from build123d import *

# Parameters (mm, degrees)
SKETCH_1_R          = 17
EXTRUDE_1_DEPTH     = 4
CUT_EXTRUDE_1_DEPTH = 2
CUT_EXTRUDE_2_REACH = 26.372
SKETCH_3_R          = 2
SKETCH_3_R_2        = 1
FILLET_1_R          = 1


with BuildPart() as part:
    # 草图1 → 凸台-拉伸1 (new body)
    with BuildSketch(Plane(origin=(0, 0, 0), x_dir=(1, 0, 0), z_dir=(0, 1, 0))):
        with Locations(Location((0, 0, 0), (0, 0, 270))):
            Circle(SKETCH_1_R)
    extrude(amount=EXTRUDE_1_DEPTH)

    # 草图2 → 切除-拉伸1 (cut)
    with BuildSketch(Plane(origin=(0, 0, 0), x_dir=(1, 0, 0), z_dir=(0, 1, 0))):
        with BuildLine():
            Line((2.5, 4.5), (2.5, -4.5))
            ThreePointArc((2.5, -4.5), (0, -7), (-2.5, -4.5))
            Line((-2.5, -4.5), (-2.5, 4.5))
            ThreePointArc((-2.5, 4.5), (0, 7), (2.5, 4.5))
        make_face()
    extrude(amount=CUT_EXTRUDE_1_DEPTH, mode=Mode.SUBTRACT)

    # 草图3 → 切除-拉伸2 (cut, up to next)
    with BuildSketch(Plane(origin=(0, 4, 0), x_dir=(1, 0, 0), z_dir=(0, 1, 0)), mode=Mode.PRIVATE) as cut_extrude_2_sk1:
        with Locations(Location((0, 11, 0), (0, 0, 270))):
            Circle(SKETCH_3_R)
    cut_extrude_2_tool1 = extrude(cut_extrude_2_sk1.sketch, amount=-CUT_EXTRUDE_2_REACH, mode=Mode.PRIVATE) & part.part
    # 草图3 → 切除-拉伸2 (cut, up to next)
    with BuildSketch(Plane(origin=(0, 4, 0), x_dir=(1, 0, 0), z_dir=(0, 1, 0)), mode=Mode.PRIVATE) as cut_extrude_2_sk2:
        with Locations(Location((-7.778174593, 7.778174593, 0), (0, 0, 270))):
            Circle(SKETCH_3_R_2)
    cut_extrude_2_tool2 = extrude(cut_extrude_2_sk2.sketch, amount=-CUT_EXTRUDE_2_REACH, mode=Mode.PRIVATE) & part.part
    # 草图3 → 切除-拉伸2 (cut, up to next)
    with BuildSketch(Plane(origin=(0, 4, 0), x_dir=(1, 0, 0), z_dir=(0, 1, 0)), mode=Mode.PRIVATE) as cut_extrude_2_sk3:
        with Locations(Location((11, 0, 0), (0, 0, 270))):
            Circle(SKETCH_3_R)
    cut_extrude_2_tool3 = extrude(cut_extrude_2_sk3.sketch, amount=-CUT_EXTRUDE_2_REACH, mode=Mode.PRIVATE) & part.part
    # 草图3 → 切除-拉伸2 (cut, up to next)
    with BuildSketch(Plane(origin=(0, 4, 0), x_dir=(1, 0, 0), z_dir=(0, 1, 0)), mode=Mode.PRIVATE) as cut_extrude_2_sk4:
        with Locations(Location((7.778174593, -7.778174593, 0), (0, 0, 270))):
            Circle(SKETCH_3_R_2)
    cut_extrude_2_tool4 = extrude(cut_extrude_2_sk4.sketch, amount=-CUT_EXTRUDE_2_REACH, mode=Mode.PRIVATE) & part.part
    add(cut_extrude_2_tool1.solids().sort_by_distance((0, 4, -11))[0], mode=Mode.SUBTRACT)
    add(cut_extrude_2_tool2.solids().sort_by_distance((-7.778175, 4, -7.778175))[0], mode=Mode.SUBTRACT)
    add(cut_extrude_2_tool3.solids().sort_by_distance((11, 4, 0))[0], mode=Mode.SUBTRACT)
    add(cut_extrude_2_tool4.solids().sort_by_distance((7.778175, 4, 7.778175))[0], mode=Mode.SUBTRACT)

    # 圆角1
    fillet_1_edges = [part.edges().sort_by_distance(p)[0] for p in [
        (0, 0, -17),
    ]]
    fillet(fillet_1_edges, radius=FILLET_1_R)


solid = part.part
Geometry check sheet. Reference: the model listing, model coordinates, mm. A direction names the side the tool comes from. Round coordinates to 2 decimals unless told otherwise and drop trailing zeros. Write each loop counter-clockwise with the first axis right and the second up, starting at its lowest first coordinate (ties: lowest second). Pieces come first, ordered by that corner, then holes. Notation, with made-up numbers: (-38, 86.25) -> (-8, 86.25) arc R20 ccw to (-8, 124.25) -> close; hole circle Ø8 at (66.25, -21). An arc over 180 degrees is marked (long way). One line per item, written item: value. Start each with the question number.
(1) Draft check along Z on faces 1 (the flat face through (0, 4, 0)), 2 (the cylindrical face through (16.855, 2.479, -2.213)), 3 (the cylindrical face through (-1.2, 2, -12.6)). Enter one of: +Z half, -Z half, draft (parallel to the pull), parting line (faces both ways), or undercut.
(2) Cross-section at C-C, the plane y = 3.45. Record the cut outline in (x, z).
(3) Cross-section at A-A, the plane x = 0. Record the cut outline in (y, z).
(4) Go/stop test with flat-tipped pins: pin 1 Ø1.5 at (x, y) = (5.5, 1.5) entering from -Z; pin 2 Ø2 at (y, z) = (1.5, 1.5) entering from -X; pin 3 Ø1.5 at (x, y) = (2.5, 1.5) entering from +Z. Record where each tip stops, or that it passes through.
(5) Scan lines: line 1 (Z direction, x = 1, y = 1.35); line 2 (X direction, y = 2.75, z = 0); line 3 (Z direction, x = -8, y = 2). Record each from-to range of solid material in increasing order. Write a range as [from, to].
(6) Access from +Z, -Z, +X, -X, +Y, -Y to the whole of each face (thin tool, end or side, straight path). Record for faces 4 (the flat face through (-2.5, 1, 0)), 5 (the cylindrical face through (-8.754, 2.028, -7.995)).
(7) Cross-section at B-B, the plane z = 0. Record the cut outline in (x, y), and give its area (3 significant figures).
Answer:
1. face 1: draft
1. face 2: parting line
1. face 3: undercut
2. outline: circle Ø34 at (0, 0); hole circle Ø2 at (-7.78, -7.78); hole circle Ø4 at (0, -11); hole circle Ø2 at (7.78, 7.78); hole circle Ø4 at (11, 0)
3. outline: (0, -16) arc R1 ccw to (1, -17) -> (4, -17) -> (4, -13) -> (0, -13) -> close; (0, -9) -> (4, -9) -> (4, 17) -> (1, 17) arc R1 ccw to (0, 16) -> (0, 7) -> (2, 7) -> (2, -7) -> (0, -7) -> close
4. pin 1: z = -16.32
4. pin 2: x = -16.99
4. pin 3: z = 16.91
5. line 1: [-16.97, -12.73], [-9.27, -6.79], [6.79, 16.97]
5. line 2: [-17, 9], [13, 17]
5. line 3: [-15, -8.75], [-6.8, 15]
6. face 4: -Y
6. face 5: +Y, -Y
7. outline: (-17, 1) arc R1 ccw to (-16, 0) -> (-2.5, 0) -> (-2.5, 2) -> (2.5, 2) -> (2.5, 0) -> (9, 0) -> (9, 4) -> (-17, 4) -> close; (13, 0) -> (16, 0) arc R1 ccw to (17, 1) -> (17, 4) -> (13, 4) -> close
7. area: 110 mm²
